Source: CAD feature listing. Evaluate the final solid. Frame: model axes, mm. A direction names the side the tool comes from. Coordinates: 2 decimals unless noted, no trailing zeros. Order: outer loops, then holes, each group sorted by start corner. A loop starts at its lowest first (then second) coordinate and runs counter-clockwise, first axis right, second up.
```python
from build123d import *

# Parameters (mm, degrees)
BOSS_EXTRUDE1_DEPTH                            = 13.8
SKETCH2_W                                      = 16.75
SKETCH2_H                                      = 23.9
CUT_EXTRUDE1_DEPTH                             = 8.25
CUT_EXTRUDE1_DEPTH_BACK                        = 4.25
SKETCH3_W                                      = 10.1
SKETCH3_H                                      = 20
CUT_EXTRUDE2_DEPTH                             = 15.5
SKETCH4_W                                      = 6.15
SKETCH4_H                                      = 20
CUT_EXTRUDE3_DEPTH                             = 12.5
FILLET1_R                                      = 1.27
CSK_FOR_M3_FLAT_HEAD_MACHINE_SCREW1_AT_2_COUNT = 2
CSK_FOR_M3_FLAT_HEAD_MACHINE_SCREW1_AT_2_PITCH = 10
CSK_FOR_M3_FLAT_HEAD_MACHINE_SCREW1_AT_3_COUNT = 2
CSK_FOR_M3_FLAT_HEAD_MACHINE_SCREW1_AT_3_PITCH = 12


with BuildPart() as part:
    # Sketch1 → Boss-Extrude1 (new body, symmetric)
    with BuildSketch(Plane.XY):
        with BuildLine():
            Line((0, -7.25), (25.75, -7.25))
            Line((25.75, -7.25), (25.75, -2.5))
            Line((25.75, -2.5), (9.954836823, 3.75))
            Line((9.954836823, 3.75), (6.204836823, 3.75))
            ThreePointArc((6.204836823, 3.75), (-6.31466547, 3.561951712), (0, -7.25))
        make_face()
    extrude(amount=BOSS_EXTRUDE1_DEPTH, both=True)

    # Sketch2 → Cut-Extrude1 (cut, two sides)
    with BuildSketch(Plane(origin=(0, 0, 0), x_dir=(1, 0, 0), z_dir=(0, 1, 0))) as cut_extrude1_sk:
        with Locations((17.375, 0)):
            Rectangle(SKETCH2_W, SKETCH2_H)
    extrude(amount=CUT_EXTRUDE1_DEPTH, mode=Mode.SUBTRACT)
    extrude(cut_extrude1_sk.sketch, amount=-CUT_EXTRUDE1_DEPTH_BACK, mode=Mode.SUBTRACT)

    # Sketch3 → Cut-Extrude2 (cut, through all)
    with BuildSketch(Plane.XZ.offset(7.25)):
        with Locations((-2.2, 0)):
            Rectangle(SKETCH3_W, SKETCH3_H)
    extrude(amount=-CUT_EXTRUDE2_DEPTH, mode=Mode.SUBTRACT)

    # Sketch4 → Cut-Extrude3 (cut, through all)
    with BuildSketch(Plane(origin=(0, -4.25, 0), x_dir=(1, 0, 0), z_dir=(0, 1, 0))):
        with Locations((5.925, 0)):
            Rectangle(SKETCH4_W, SKETCH4_H)
    extrude(amount=CUT_EXTRUDE3_DEPTH, mode=Mode.SUBTRACT)

    # Fillet1
    fillet1_edges = [part.edges().sort_by_distance(p)[0] for p in [
        (25.75, -2.5, -12.875),
        (25.75, -2.5, 12.875),
    ]]
    fillet(fillet1_edges, radius=FILLET1_R)

    # Sketch6 → CSK for M3 Flat Head Machine Screw1 (revolve, cut)
    with BuildSketch(Plane(origin=(21.75, -4.25, -6), x_dir=(0, 0, 1), z_dir=(1, 0, 0))):
        Polygon((0, 0), (0, 3), (1.7, 3), (1.7, 1.45), (3.15, 0), align=None)
    csk_for_m3_flat_head_machine_screw1 = revolve(axis=Axis((21.75, 2.1, -6), (0, -1, 0)), mode=Mode.SUBTRACT)

    # CSK for M3 Flat Head Machine Screw1 at 2: CSK for M3 Flat Head Machine Screw1 ×2
    with Locations(*[Vector(-0.8, 0, 0.6) * (i * CSK_FOR_M3_FLAT_HEAD_MACHINE_SCREW1_AT_2_PITCH) for i in range(1, CSK_FOR_M3_FLAT_HEAD_MACHINE_SCREW1_AT_2_COUNT)]):
        add(csk_for_m3_flat_head_machine_screw1, mode=Mode.SUBTRACT)

    # CSK for M3 Flat Head Machine Screw1 at 3: CSK for M3 Flat Head Machine Screw1 ×2
    with Locations(*[(0, 0, i * CSK_FOR_M3_FLAT_HEAD_MACHINE_SCREW1_AT_3_PITCH) for i in range(1, CSK_FOR_M3_FLAT_HEAD_MACHINE_SCREW1_AT_3_COUNT)]):
        add(csk_for_m3_flat_head_machine_screw1, mode=Mode.SUBTRACT)


solid = part.part
```
1. Draft query along Z for faces 1 (the face through (25.75, -6, 0)), 2 (the face through (15, -1, 11.95)), 3 (the face through (5, -2, -13.8)). Return one class per face: released by +Z, released by -Z, zero draft, split by the parting line, or undercut.
Findings:
face 1: zero draft
face 2: undercut
face 3: released by -Z
2. Ray query, line 1 (Z direction, x = 21.75, y = -6.8); line 2 (X direction, y = -6.75, z = 6); line 3 (Z direction, x = 13.75, y = -6.8). Return the intervals inside material, ascending.
Findings:
line 1: z = -13.8 to -7.7, -4.3 to 4.3, 7.7 to 13.8
line 2: x = 2.85 to 20.05, 23.45 to 25.75
line 3: z = -13.8 to -1.7, 1.7 to 13.8
3. Section query A-A on z = 0. Return loops of the section in (x, y), plus the area to 3 significant figures.
Findings:
outline: (2.85, -7.25) - (12.05, -7.25) - (12.05, -5.7) - (10.6, -4.25) - (2.85, -4.25) - close; (15.45, -7.25) - (25.75, -7.25) - (25.75, -4.25) - (16.9, -4.25) - (15.45, -5.7) - close
area: 56.4 mm2
4. Section query B-B on y = 0. Return loops of the section in (x, z).
Findings:
outline: (-7.25, -13.8) - (19.43, -13.8) - (19.43, -11.95) - (9, -11.95) - (9, -10) - (-7.25, -10) - close; (-7.25, 10) - (9, 10) - (9, 11.95) - (19.43, 11.95) - (19.43, 13.8) - (-7.25, 13.8) - close
5. Section query C-C on x = 21.75. Return loops of the section in (y, z).
Findings:
outline: (-7.25, -13.8) - (-0.92, -13.8) - (-0.92, -11.95) - (-4.25, -11.95) - (-4.25, -9.15) - (-5.7, -7.7) - (-7.25, -7.7) - close; (-7.25, -4.3) - (-5.7, -4.3) - (-4.25, -2.85) - (-4.25, 2.85) - (-5.7, 4.3) - (-7.25, 4.3) - close; (-7.25, 7.7) - (-5.7, 7.7) - (-4.25, 9.15) - (-4.25, 11.95) - (-0.92, 11.95) - (-0.92, 13.8) - (-7.25, 13.8) - close
6. Access query for faces 4 (the face through (8, 3.75, 12)), 5 (the face through (12.064, -6.464, -0.221)), 6 (the face through (9, 0, -11)), 7 (the face through (2.85, -6, 0)), 8 (the face through (16, -7.25, 0)). Directions: +Z, -Z, +X, -X, +Y, -Y. A direction counts if a zero-diameter tool reaches every point of the face in a straight line with its end or side. Return the directions, or none.
Findings:
face 4: +Z, -Z, +X, +Y
face 5: +Y, -Y
face 6: +X, +Y
face 7: -X, +Y, -Y
face 8: +Z, -Z, +X, -X, -Y
7. Section query D-D on x = 5. Return loops of the section in (y, z).
Findings:
outline: (-7.25, -13.8) - (5.25, -13.8) - (5.25, -10) - (-4.25, -10) - (-4.25, 10) - (5.25, 10) - (5.25, 13.8) - (-7.25, 13.8) - close
8. Pin query (flat end, axial travel): P1, Ø5.5, axis at x = 21.75, z = -6, coming from the -Y side; P2, Ø0.6, axis at y = -0.5, z = 11.5, coming from the +X side; P3, Ø2.5, axis at y = -5.5, z = 0, coming from the -X side; P4, Ø1.1, axis at x = 7.5, z = -13, coming from the +Y side. Return the tip coordinate at first contact, or that it passes through.
Findings:
P1: stops at y = -7.25
P2: stops at x = 9
P3: stops at x = 2.85
P4: stops at y = 3.75
